The listing builds one solid part. Answer for the finished solid, in the listing's coordinates (mm). A direction names the side the tool comes from. Give positions to 0.01 mm unless a question says otherwise; leave off trailing zeros. Write each loop counter-clockwise with the first axis right and the second up, starting at its lowest first coordinate (ties: lowest second). Pieces come first, ordered by that corner, then holes. Notation, with made-up numbers: (18, 32) - (69, 32) arc R37 cw to (69, 69) - close; hole circle Ø4 at (85, 74.5). An arc over 180 degrees is marked (long way). One line per question, with ' | ' between items. Start each with the question number.
1. A cutting plane is placed at D-D (y = 1.75). Determine the outline of the cut face in (x, z).
2. A cutting plane is placed at A-A (y = 3.5). Determine the outline of the cut face in (x, z), then the cut area to 3 significant figures.
3. The mould has two halves that part along Z. Classify faces 1 (the face through (2.5, 0.5, -10)), 2 (the face through (3, 7, -3)), 3 (the face through (2, 3, 0)), 4 (the face through (2.5, 6, -2.5)): +Z half, -Z half, draft (parallel to the pull), parting line (faces both ways), or undercut.
4. Find the intervals of material crossed by L1, parallel to X at y = 2.75, z = -2.5; L2, parallel to Z at x = 1.85, y = 4; L3, parallel to X at y = 1.75, z = -4.5, in increasing order. Write a range as from..to.
5. Given P1, Ø0.8, axis at x = 2.5, z = -2.5, coming from the -Y side, flat-ended and moving along its own axis, determine where the tip first touches the part or whether it passes through.
6. A cutting plane is placed at B-B (z = -2.5). Determine the outline of the cut face in (x, y).
7. A cutting plane is placed at C-C (x = 2.5). Determine the outline of the cut face in (y, z).
8. For faces 5 (the face through (1, 6, -1)), 6 (the face through (2, 0, -5)), 7 (the face through (2.883, 2.535, -4.076)), determine the directions among +Z, -Z, +X, -X, +Y, -Y from which every point of the face is accessible in a straight line to the end or side of a thin tool.
```python
from build123d import *

# Parameters (mm, degrees)
BOSS_EXTRUDE2_DEPTH = 5
CUT_EXTRUDE1_DEPTH  = 4
BOSS_EXTRUDE3_DEPTH = 1
CUT_EXTRUDE2_REACH  = 14.689
SKETCH4_R           = 0.75
SKETCH4_4_R         = 1.5
SKETCH4_4_R_2       = 0.75
BOSS_EXTRUDE6_DEPTH = 1
SKETCH6_R           = 1
BOSS_EXTRUDE7_DEPTH = 5


with BuildPart() as part:
    # Sketch3 → Boss-Extrude2 (new body)
    with BuildSketch(Plane(origin=(0, 0, 0), x_dir=(0, 0, -1), z_dir=(1, 0, 0))):
        Polygon((5, 5), (4, 6), (1, 6), (0, 6), (0, 0), (1, 0), (1, 5), align=None)
        Polygon((9, 1), (5, 5), (1, 5), (1, 0), (9, 0), align=None)
        Polygon((10, 1), (5, 6), (4, 6), (5, 5), (9, 1), (9, 0), (10, 0), align=None)
    extrude(amount=BOSS_EXTRUDE2_DEPTH)

    # Sketch3<5> → Cut-Extrude1 (cut)
    with BuildSketch(Plane(origin=(0, 0, 0), x_dir=(0, 0, -1), z_dir=(1, 0, 0))):
        Polygon((9, 1), (5, 5), (1, 5), (1, 0), (9, 0), align=None)
    extrude(amount=CUT_EXTRUDE1_DEPTH, mode=Mode.SUBTRACT)

    # Sketch3<6> → Boss-Extrude3 (add)
    with BuildSketch(Plane(origin=(0, 0, 0), x_dir=(0, 0, -1), z_dir=(1, 0, 0))):
        Polygon((9, 1), (5, 5), (1, 5), (1, 0), (9, 0), align=None)
    extrude(amount=BOSS_EXTRUDE3_DEPTH)

    # Sketch4 → Cut-Extrude2 (cut, up to next)
    with BuildSketch(Plane(origin=(0, 6, 0), x_dir=(1, 0, 0), z_dir=(0, 1, 0)), mode=Mode.PRIVATE) as cut_extrude2_sk1:
        with Locations(Location((2.5, 2.5, 0), (0, 0, 270))):
            Circle(SKETCH4_R)
    cut_extrude2_tool1 = extrude(cut_extrude2_sk1.sketch, amount=-CUT_EXTRUDE2_REACH, mode=Mode.PRIVATE) & part.part
    add(cut_extrude2_tool1.solids().sort_by_distance((2.5, 6, -2.5))[0], mode=Mode.SUBTRACT)

    # Sketch4<4> → Boss-Extrude6 (add)
    with BuildSketch(Plane(origin=(0, 6, 0), x_dir=(1, 0, 0), z_dir=(0, 1, 0))):
        with Locations(Location((2.5, 2.5, 0), (0, 0, 270))):
            Circle(SKETCH4_4_R)
        with Locations(Location((2.5, 2.5, 0), (0, 0, 270))):
            Circle(SKETCH4_4_R_2, mode=Mode.SUBTRACT)
        with Locations(Location((2.5, 2.5, 0), (0, 0, 270))):
            Circle(SKETCH4_4_R_2)
    extrude(amount=BOSS_EXTRUDE6_DEPTH)

    # Sketch6 → Boss-Extrude7 (add)
    with BuildSketch(Plane(origin=(0, 5, 0), x_dir=(-1, 0, 0), z_dir=(0, -1, 0))):
        with Locations(Location((-2.5, 5, 0), (0, 0, 270))):
            Circle(SKETCH6_R)
    extrude(amount=BOSS_EXTRUDE7_DEPTH)


solid = part.part
```
Determined:
1) outline: (0, -9.25) - (5, -9.25) - (5, 0) - (0, 0) - close; circle Ø2 at (2.5, -5); hole (1, -8.25) - (4, -8.25) - (4, -1) - (1, -1) - close
2) outline: (0, -7.5) - (5, -7.5) - (5, 0) - (0, 0) - close; circle Ø2 at (2.5, -5); hole (1, -6.5) - (4, -6.5) - (4, -1) - (1, -1) - close | area: 24.1 mm2
3) face 1: -Z half | face 2: draft | face 3: +Z half | face 4: undercut
4) L1: 0..1, 4..5 | L2: -7..-6, -5.76..-4.24, -1..0 | L3: 0..1, 1.63..3.37, 4..5
5) P1: y = 6
6) outline: (0, 0) - (1, 0) - (1, 5) - (1.75, 5) - (1.75, 6) - (3.25, 6) - (3.25, 5) - (4, 5) - (4, 0) - (5, 0) - (5, 6) - (4, 6) - (4, 7) - (1, 7) - (1, 6) - (0, 6) - close
7) outline: (0, -10) - (1, -10) - (6, -5) - (6, -4) - (7, -4) - (7, -1) - (6, -1) - (6, 0) - (0, 0) - (0, -1) - (5, -1) - (5, -1.75) - (6, -1.75) - (6, -3.25) - (5, -3.25) - (5, -4) - (0, -4) - (0, -6) - (4, -6) - (1, -9) - (0, -9) - close
8) face 5: +Y | face 6: +Z, -Z, +X, -X, -Y | face 7: -Y
